Autodesk Inventor part; units mm, degrees
ref_plane "YZ Plane" through (0, 0, 0) normal (1, 0, 0) x (0, 1, 0)
ref_plane "XZ Plane" through (0, 0, 0) normal (0, 1, 0) x (-1, 0, 0)
ref_plane "XY Plane" through (0, 0, 0) normal (0, 0, 1) x (1, 0, 0)
sketch "Sketch1" plane through (0, 0, 0) normal (1, 0, 0) x (0, 1, 0)
  line L0 (0, 0) -> (0, 60.75)
  line L1 (0, 60.75) -> (25, 60.75)
  line L2 (25, 60.75) -> (25, 57.75)
  line L3 (25, 57.75) -> (3.5, 57.75)
  line L4 (3.5, 57.75) -> (3.5, 52.75)
  line L5 (3.5, 52.75) -> (25, 52.75)
  line L6 (25, 52.75) -> (25, 49.75)
  line L7 (25, 49.75) -> (3.5, 49.75)
  line L8 (3.5, 49.75) -> (3.5, 0)
  line L9 (3.5, 0) -> (0, 0)
  line L10 (25, 57.75) -> (25, 52.75) construction
  line L11 (3.5, 55.25) -> (25, 55.25) construction
  line L12 (-5, 0) -> (30, 0)
  dimension "d1" = 25
  dimension "d2" = 3
  dimension "d4" = 5
  dimension "d7" = 3.5
  dimension "d8" = 55.25
  dimension "d9" = 3.5
revolve "Revolution1" add sketch "Sketch1" angle 360 about axis through (0, -10, 0) along (0, 1, 0)
sketch "Sketch2" plane through (0, 3.5, 0) normal (0, 1, 0) x (1, 0, 0)
  circle A0 centre (0, 0) radius 17.5
  dimension "d11" = 35
extrude "Extrusion1" cut sketch "Sketch2" against normal blind 40
properties part number "Base"
CAD build for the part. Positions are in the model's coordinates, mm. A direction names the side the tool comes from. Round coordinates to 2 decimals unless told otherwise and drop trailing zeros. Write each loop counter-clockwise with the first axis right and the second up, starting at its lowest first coordinate (ties: lowest second). Pieces come first, ordered by that corner, then holes. Notation, with made-up numbers: (69.25, 17) - (79.25, 17) arc R14 ccw to (79.25, 37) - close; hole circle Ø7 at (3, -5.5). An arc over 180 degrees is marked (long way). Return JSON: item names as keys, results as strings. Group by question number.
Item 1: Band-saw the part on B-B on z = 0. List the corners of the cut face in (x, y), plus the area to 3 significant figures.
Item 2: 3-axis set-ups, long thin cutter, end or side, ignore diameter. For faces 4 (the face through (-13.887, 1.774, 10.648)), 5 (the face through (30.27, 14.1, -39.48)): which of +Z, -Z, +X, -X, +Y, -Y reach the whole face in a straight line?
Item 3: Probe probe 1 along X at (y, z) = (18.5, 0); probe 2 along Z at (x, y) = (37.5, 16); probe 3 along X at (y, z) = (23.75, -12.5). List the from-to ranges inside material, lowest first.
Item 4: Flat gauge pins, fed straight in: pin 1 Ø3 at (y, z) = (20.5, -30.5) entering from +X; pin 2 Ø1.5 at (x, z) = (21.5, 21) entering from +Y; pin 3 Ø1.5 at (y, z) = (13, 17) entering from +X. Where does each tip first touch, or does it go through?
Item 5: Band-saw the part on D-D on z = -37. List the corners of the cut face in (x, y).
Item 6: Mould opens along Z. For faces 1 (the face through (-13, 0, 13)), 2 (the face through (-21, 3.5, -1)), 3 (the face through (18.248, 12.675, 57.945)) say: +Z half, -Z half, draft (parallel to the pull), parting line (faces both ways), or undercut.
Item 7: Band-saw the part on C-C on y = 5. List the corners of the cut face in (x, z), plus the area to 3 significant figures.
Item 8: Band-saw the part on A-A on x = 0. List the corners of the cut face in (y, z), plus the area to 3 significant figures.
Resolved:
{
 "1": {"outline": "(-60.75, 0) - (-17.5, 0) - (-17.5, 3.5) - (-49.75, 3.5) - (-49.75, 25) - (-52.75, 25) - (-52.75, 3.5) - (-57.75, 3.5) - (-57.75, 25) - (-60.75, 25) - close; (17.5, 0) - (60.75, 0) - (60.75, 25) - (57.75, 25) - (57.75, 3.5) - (52.75, 3.5) - (52.75, 25) - (49.75, 25) - (49.75, 3.5) - (17.5, 3.5) - close", "area": "561 mm²"},
 "2": {"face 4": "+Y, -Y", "face 5": "+Y"},
 "3": {"probe 1": "x = -60.75 to -57.75, -52.75 to -49.75, 49.75 to 52.75, 57.75 to 60.75", "probe 2": "z = -47.79 to -43.92, -37.1 to -32.69, 32.69 to 37.1, 43.92 to 47.79", "probe 3": "x = -59.45 to -56.38, -51.25 to -48.15, 48.15 to 51.25, 56.38 to 59.45"},
 "4": {"pin 1": "stops at x = 53.38", "pin 2": "stops at y = 3.5", "pin 3": "stops at x = 58.54"},
 "5": {"outline": "(-48.18, 0) - (48.18, 0) - (48.18, 25) - (44.34, 25) - (44.34, 3.5) - (37.6, 3.5) - (37.6, 25) - (33.26, 25) - (33.26, 3.5) - (-33.26, 3.5) - (-33.26, 25) - (-37.6, 25) - (-37.6, 3.5) - (-44.34, 3.5) - (-44.34, 25) - (-48.18, 25) - close"},
 "6": {"face 1": "draft", "face 2": "undercut", "face 3": "parting line"},
 "7": {"outline": "circle Ø121.5 at (0, 0); circle Ø105.5 at (0, 0); hole circle Ø115.5 at (0, 0); hole circle Ø99.5 at (0, 0)", "area": "2,080 mm²"},
 "8": {"outline": "(0, -60.75) - (25, -60.75) - (25, -57.75) - (3.5, -57.75) - (3.5, -52.75) - (25, -52.75) - (25, -49.75) - (3.5, -49.75) - (3.5, -17.5) - (0, -17.5) - close; (0, 17.5) - (3.5, 17.5) - (3.5, 49.75) - (25, 49.75) - (25, 52.75) - (3.5, 52.75) - (3.5, 57.75) - (25, 57.75) - (25, 60.75) - (0, 60.75) - close", "area": "561 mm²"}
}
